```python
from build123d import *

# Parameters (mm, degrees)
CROQUIS2_R            = 4
CORTAR_EXTRUIR1_DEPTH = 81.132952023
CHAFL_N1_SIZE         = 1


with BuildPart() as part:
    # Croquis1 → Revolución1 (revolve)
    with BuildSketch(Plane.XY, mode=Mode.PRIVATE) as revoluci_n1_sk:
        Polygon((0, 22.25), (9.5, 22.25), (9.5, 10), (41.2, 10), (41.2, 15.5), (31.7, 15.5), (31.7, 18), (31.7, 19), (23.7, 19), (23.7, 18), (17, 18), (17, 28.5), (3.5, 28.5), (3.5, 50), (0, 50), align=None)
    revolve(revoluci_n1_sk.sketch.rotate(Axis((-60.102579917, 0, 0), (1, 0, 0)), 90), axis=Axis((-60.102579917, 0, 0), (1, 0, 0)))

    # Croquis2 → Cortar-Extruir1 (cut, through all)
    with BuildSketch(Plane(origin=(3.5, 0, 0), x_dir=(0, 0, -1), z_dir=(1, 0, 0))):
        with Locations((0, 43)):
            Circle(CROQUIS2_R)
        with Locations((30.405591591, 30.405591591)):
            Circle(CROQUIS2_R)
        with Locations((43, 0)):
            Circle(CROQUIS2_R)
        with Locations((30.405591591, -30.405591591)):
            Circle(CROQUIS2_R)
        with Locations((0, -43)):
            Circle(CROQUIS2_R)
        with Locations((-30.405591591, -30.405591591)):
            Circle(CROQUIS2_R)
        with Locations((-43, 0)):
            Circle(CROQUIS2_R)
        with Locations((-30.405591591, 30.405591591)):
            Circle(CROQUIS2_R)
    extrude(amount=-CORTAR_EXTRUIR1_DEPTH, mode=Mode.SUBTRACT)

    # Chaflán1
    chafl_n1_edges = [part.edges().sort_by_distance(p)[0] for p in [
        (23.7, 0, -19),
        (31.7, 0, -19),
    ]]
    chamfer(chafl_n1_edges, length=CHAFL_N1_SIZE - 0.0001)  # a hair under: the kernel refuses the full size


solid = part.part
```
Here's how the part is built. I have some questions about the finished solid (model axes, mm). A direction names the side the tool comes from. Coordinates: 2 decimals unless noted, no trailing zeros. Order: outer loops, then holes, each group sorted by start corner. A loop starts at its lowest first (then second) coordinate and runs counter-clockwise, first axis right, second up.
1) Imagine slicing it at C-C on x = 29. List the corners of the cut face in (y, z) for me, and give its area (3 significant figures).
2) Will these pins go through, and if not, where does the flat tip stop? pin 1 (10.5 mm diameter, centred on y = 0, z = 43, fed in from +X); pin 2 (4 mm diameter, centred on x = 26, y = -16, fed in from +Z); pin 3 (6 mm diameter, centred on y = 15, z = 12, fed in from +X).
3) Imagine slicing it at D-D on z = 0. State how many separate pieces and enclosed holes the cut face has, and give its area (3 significant figures).
4) I need wall thicknesses on line 1 (Y direction, x = 5, z = 0); line 2 (X direction, y = -41.5, z = 21); line 3 (X direction, y = 1, z = -28). Which ranges of each line are inside material? Lowest first, please.
5) We'd pull the mould along Y, two halves only. Please class faces 4 (the face through (41.2, 3, -10)), 5 (the face through (1.77, -31.94, -34.1)), 6 (the face through (10.156, 25.284, 13.151)): +Y half, -Y half, draft (parallel to the pull), parting line (faces both ways), or undercut.
6) Which directions (+Z, -Z, +X, -X, +Y, -Y) give clear straight access to the entire face, cutting with the end or side of a thin tool? Please do faces 1 (the face through (20.303, -12.165, -13.267)), 2 (the face through (36.384, -15.368, -2.018)), 3 (the face through (9.5, 10, 5)).
7) Imagine slicing it at A-A on z = 43. List the corners of the cut face in (x, y) for me.
Response values:
1. outline: circle Ø38 at (0, 0); hole circle Ø20 at (0, 0)
1. area: 820 mm2
2. pin 1: stops at x = 3.5
2. pin 2: stops at z = 12.85
2. pin 3: stops at x = 31.7
3. separate pieces: 4
3. enclosed holes: 0
3. area: 844 mm2
4. line 1: y = -28.5 to -22.25, 22.25 to 28.5
4. line 2: x = 0 to 3.5
4. line 3: x = 0 to 17
5. face 4: draft
5. face 5: undercut
5. face 6: parting line
6. face 1: none
6. face 2: +X
6. face 3: -X
7. outline: (0, -25.51) - (3.5, -25.51) - (3.5, -4) - (0, -4) - close; (0, 4) - (3.5, 4) - (3.5, 25.51) - (0, 25.51) - close
